Input: part model. Units: mm. Frame: model coordinates. Face numbers are marked on the shaded views. Round coordinates to 2 decimals unless told otherwise and drop trailing zeros. Order: outer loops, then holes, each group sorted by start corner. A loop starts at its lowest first (then second) coordinate and runs counter-clockwise, first axis right, second up.
Item 1: Cut plane C-C on y = -2.9. Output: boundary loops of the cut face in (x, z).
Item 2: Cut plane A-A on z = 0. Output: boundary loops of the cut face in (x, y), then the cut area to 3 significant figures.
Item 3: Mould query, pull axis X, two halves, no side actions, for the marked faces 1, 2 and 3. Classes: released by +X, released by -X, zero draft, split by the parting line, or undercut.
Item 4: First-contact query: pin 1 (2 mm diameter, centred on x = -4.5, y = -0.5, fed in from -Z); pin 2 (5 mm diameter, centred on x = 0, z = -2, fed in from -Y); pin 3 (1.5 mm diameter, centred on x = 4, y = -1.5, fed in from +Z). Flat tips, straight axial feed; report the tip coordinate or a pass-through.
Item 5: Cut plane D-D on z = 6.5. Output: boundary loops of the cut face in (x, y).
Item 6: Line query: L1, parallel to Z at x = 0, y = -1.9; L2, parallel to Z at x = 0, y = -1; L3, parallel to Y at x = -8.5, z = 4. Output: solid intervals per line, ascending.
Item 7: Cut plane B-B on x = 0. Output: boundary loops of the cut face in (y, z), then the cut area to 3 significant figures.
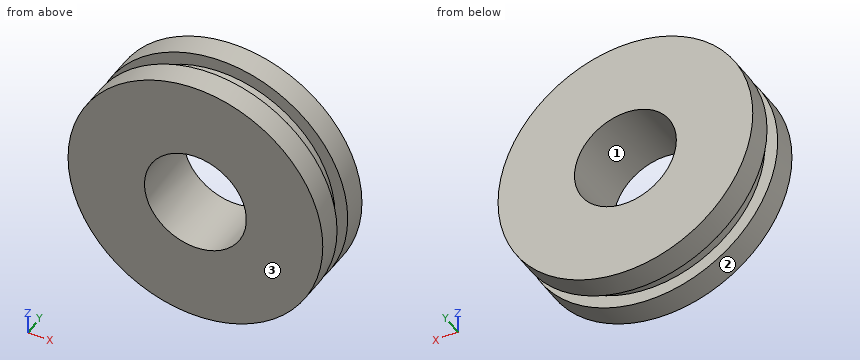
```python
from build123d import *

# Parameters (mm, degrees)
F0_R     = 9
F1_DEPTH = 1.5
F2_R     = 10
F3_DEPTH = 2
F4_R     = 10
F5_DEPTH = 2
F7_D     = 8


with BuildPart() as f1:
    # F0 (on Front) → F1 (new body)
    with BuildSketch(Plane.XZ):
        Circle(F0_R)
    extrude(amount=F1_DEPTH)

    # F2 (on face) → F3 (join)
    with BuildSketch(Plane.XZ.offset(1.5)):
        Circle(F2_R)
    extrude(amount=F3_DEPTH)

    # F4 (on face) → F5 (join)
    with BuildSketch(Plane(origin=(0, 0, 0), x_dir=(-1, 0, 0), z_dir=(0, 1, 0))):
        Circle(F4_R)
    extrude(amount=F5_DEPTH)

    # F7 (through all)
    with Locations(Plane.XZ.offset(3.5)):
        with Locations((0, 0)):
            Hole(F7_D / 2)


solid = f1.part
```
From the geometry:
1. outline: circle Ø20 at (0, 0); hole circle Ø8 at (0, 0)
2. outline: (-10, -3.5) - (-4, -3.5) - (-4, 2) - (-10, 2) - (-10, 0) - (-9, 0) - (-9, -1.5) - (-10, -1.5) - close; (4, -3.5) - (10, -3.5) - (10, -1.5) - (9, -1.5) - (9, 0) - (10, 0) - (10, 2) - (4, 2) - close
2. area: 63.0 mm2
3. face 1: undercut
3. face 2: split by the parting line
3. face 3: zero draft
4. pin 1: stops at z = -9.32
4. pin 2: stops at y = -3.5
4. pin 3: stops at z = 9.46
5. outline: (-7.6, -3.5) - (7.6, -3.5) - (7.6, -1.5) - (6.22, -1.5) - (6.22, 0) - (7.6, 0) - (7.6, 2) - (-7.6, 2) - (-7.6, 0) - (-6.22, 0) - (-6.22, -1.5) - (-7.6, -1.5) - close
6. L1: z = -10 to -4, 4 to 10
6. L2: z = -9 to -4, 4 to 9
6. L3: y = -3.5 to -1.5, 0 to 2
7. outline: (-3.5, -10) - (-1.5, -10) - (-1.5, -9) - (0, -9) - (0, -10) - (2, -10) - (2, -4) - (-3.5, -4) - close; (-3.5, 4) - (2, 4) - (2, 10) - (0, 10) - (0, 9) - (-1.5, 9) - (-1.5, 10) - (-3.5, 10) - close
7. area: 63.0 mm2
